For this review, take the finished solid that the model builds, in its own axes (mm). A direction names the side the tool comes from. Coordinates: 2 decimals unless noted, no trailing zeros. Write each loop counter-clockwise with the first axis right and the second up, starting at its lowest first coordinate (ties: lowest second). Pieces come first, ordered by that corner, then holes.
```python
from build123d import *

# Parameters (mm, degrees)
F1_DEPTH = 870
F6_DEPTH = 7
F7_DEPTH = 7


with BuildPart() as f1:
    # F0 (on Top) → F1 (new body)
    with BuildSketch(Plane.XY):
        with BuildLine():
            Line((-50, 0), (0, 0))
            Line((0, 0), (0, 50))
            ThreePointArc((0, 50), (-3.535534, 48.535534), (-5, 45))
            Line((-5, 45), (-5, 10))
            ThreePointArc((-5, 10), (-6.464466, 6.464466), (-10, 5))
            Line((-10, 5), (-45, 5))
            ThreePointArc((-45, 5), (-48.535534, 3.535534), (-50, 0))
        make_face()
    extrude(amount=F1_DEPTH)

    # F3 (on face) + F4 (on face) → F6 (cut)
    with BuildSketch(Plane.YZ):
        Polygon((0, 820), (50, 870), (0, 870), align=None)
    with BuildSketch(Plane.YZ):
        Polygon((0, 0), (50, 0), (0, 50), align=None)
    extrude(amount=-F6_DEPTH, mode=Mode.SUBTRACT)

    # F2 (on face) → F7 (cut)
    with BuildSketch(Plane.XZ):
        Polygon((0, 870), (-50, 870), (0, 820), align=None)
        Polygon((0, 50), (-50, 0), (0, 0), align=None)
    extrude(amount=-F7_DEPTH, mode=Mode.SUBTRACT)


solid = f1.part
```
Q1. Add section A-A (z = 119). State the section outline as (x, y) points, then the cut area to 3 significant figures.
Ans:
outline: (-50, 0) - (0, 0) - (0, 50) arc R5 ccw to (-5, 45) - (-5, 10) arc R5 cw to (-10, 5) - (-45, 5) arc R5 ccw to start
area: 470 mm2
Q2. Tool access review of faces 1 (the flat face through (-29, 2, 849)), 2 (the flat face through (-5, 28, 429)): name each direction out of +Z, -Z, +X, -X, +Y, -Y from which nothing blocks a thin tool from reaching the whole face with its end or side.
Ans:
face 1: +Z, +X, +Y, -Y
face 2: +Z, -Z, -X, +Y
Q3. Clearance check with flat-ended pins moving along their axes: pin 1 Ø1.5 at (y, z) = (36.5, 122) entering from +X; pin 2 Ø6.5 at (y, z) = (2.5, 825) entering from +X; pin 3 Ø10 at (y, z) = (19.5, 710.5) entering from -X; pin 4 Ø12 at (x, y) = (-7, 38.5) entering from -Z. State where each tip first meets the part, or that it passes through.
Ans:
pin 1: stops at x = 0
pin 2: stops at x = -1.75
pin 3: stops at x = -5
pin 4: stops at z = 5.84
Q4. For probe 1 along X at (y, z) = (6.5, 354.5); probe 2 along Y at (x, z) = (-18.5, 73); probe 3 along X at (y, z) = (41, 733), list the stretches that pass through material, from the lowest coordinate up.
Ans:
probe 1: x = -6.43 to 0
probe 2: y = 0 to 5
probe 3: x = -5 to 0
Q5. Add section C-C (y = 34). State the section outline as (x, z) points.
Ans:
outline: (-5, 16) - (0, 16) - (0, 854) - (-5, 854) - close
Q6. Add section B-B (x = -23). State the section outline as (y, z) points.
Ans:
outline: (0, 27) - (5, 27) - (5, 843) - (0, 843) - close
